```python
from build123d import *

# Parameters (mm, degrees)
F0_R     = 44.45
F0_R_2   = 36.51
F1_DEPTH = 55
F2_R     = 44.45
F2_R_2   = 41.2
F3_DEPTH = 10
F4_R     = 44.45
F4_R_2   = 41.45
F5_DEPTH = 5
F4_R_3   = 37.5
F4_R_4   = 36.51
F6_DEPTH = 37


with BuildPart() as f1:
    # F0 (on Front) → F1 (new body)
    with BuildSketch(Plane.XZ):
        Circle(F0_R)
        Circle(F0_R_2, mode=Mode.SUBTRACT)
    extrude(amount=F1_DEPTH)

    # F2 (on face) → F3 (cut)
    with BuildSketch(Plane.XZ.offset(55)):
        Circle(F2_R)
        Circle(F2_R_2, mode=Mode.SUBTRACT)
    extrude(amount=-F3_DEPTH, mode=Mode.SUBTRACT)

    # F4 (on face) → F5 (cut)
    with BuildSketch(Plane(origin=(0, 0, 0), x_dir=(-1, 0, 0), z_dir=(0, 1, 0))):
        Circle(F4_R)
        Circle(F4_R_2, mode=Mode.SUBTRACT)
    extrude(amount=-F5_DEPTH, mode=Mode.SUBTRACT)

    # F4 (on face) → F6 (cut)
    with BuildSketch(Plane(origin=(0, 0, 0), x_dir=(-1, 0, 0), z_dir=(0, 1, 0))):
        Circle(F4_R_3)
        Circle(F4_R_4, mode=Mode.SUBTRACT)
    extrude(amount=-F6_DEPTH, mode=Mode.SUBTRACT)


solid = f1.part
```
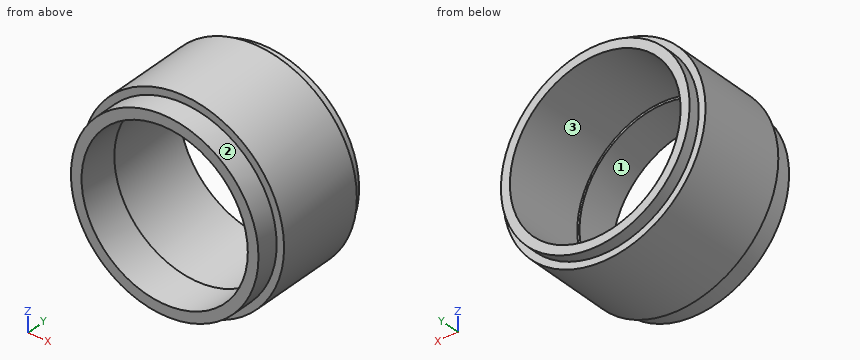
Could you check a few things on this model? Use its own coordinates, in mm. Face numbers are marked on the shaded views. A direction names the side the tool comes from. Give positions to 0.01 mm unless a question says otherwise; leave off trailing zeros. Order: outer loops, then holes, each group sorted by start corner. A loop starts at its lowest first (then second) coordinate and runs counter-clockwise, first axis right, second up.
Q1. Suppose I cut it at C-C, the plane y = -15. Write out the boundary of the cut face in (x, z), and give its area (3 significant figures).
Q2. I'm going to push flat-ended pins straight in: P1, Ø6, axis at x = 15, y = -34, coming from the +Z side; P2, Ø10, axis at y = -32.5, z = 17, coming from the +X side; P3, Ø8, axis at x = 21.5, y = -26.5, coming from the +Z side; P4, Ø6, axis at x = 32, z = -17, coming from the +Y side. Where does each tip first touch, or does it pass through?
Q3. Suppose I cut it at A-A, the plane x = 0. Write out the boundary of the cut face in (y, z).
Q4. For the marked faces 1, 2 and 3, which set-ups out of +Z, -Z, +X, -X, +Y, -Y let a thin tool reach every point of the face, with its end or its side?
Q5. If I drill on line 1 along Z through (x, y) = (0, -17.5); line 2 along Z through (x, y) = (0, -41); line 3 along X through (y, z) = (-36.5, 2.5), over which ranges is the centre line in solid material (lowest first)?
Q6. Suppose I cut it at B-B, the plane z = 0. Write out the boundary of the cut face in (x, y).
Solution:
1. outline: circle Ø88.9 at (0, 0); hole circle Ø75 at (0, 0)
1. area: 1,790 mm2
2. P1: stops at z = 42.8
2. P2: stops at x = 42.8
2. P3: stops at z = 40.86
2. P4: stops at y = 0
3. outline: (-55, -41.2) - (-45, -41.2) - (-45, -44.45) - (-5, -44.45) - (-5, -41.45) - (0, -41.45) - (0, -37.5) - (-37, -37.5) - (-37, -36.51) - (-55, -36.51) - close; (-55, 36.51) - (-37, 36.51) - (-37, 37.5) - (0, 37.5) - (0, 41.45) - (-5, 41.45) - (-5, 44.45) - (-45, 44.45) - (-45, 41.2) - (-55, 41.2) - close
4. face 1: +Y, -Y
4. face 2: -Y
4. face 3: +Y
5. line 1: z = -44.45 to -37.5, 37.5 to 44.45
5. line 2: z = -44.45 to -36.51, 36.51 to 44.45
5. line 3: x = -44.38 to -37.42, 37.42 to 44.38
6. outline: (-44.45, -45) - (-41.2, -45) - (-41.2, -55) - (-36.51, -55) - (-36.51, -37) - (-37.5, -37) - (-37.5, 0) - (-41.45, 0) - (-41.45, -5) - (-44.45, -5) - close; (36.51, -55) - (41.2, -55) - (41.2, -45) - (44.45, -45) - (44.45, -5) - (41.45, -5) - (41.45, 0) - (37.5, 0) - (37.5, -37) - (36.51, -37) - close
